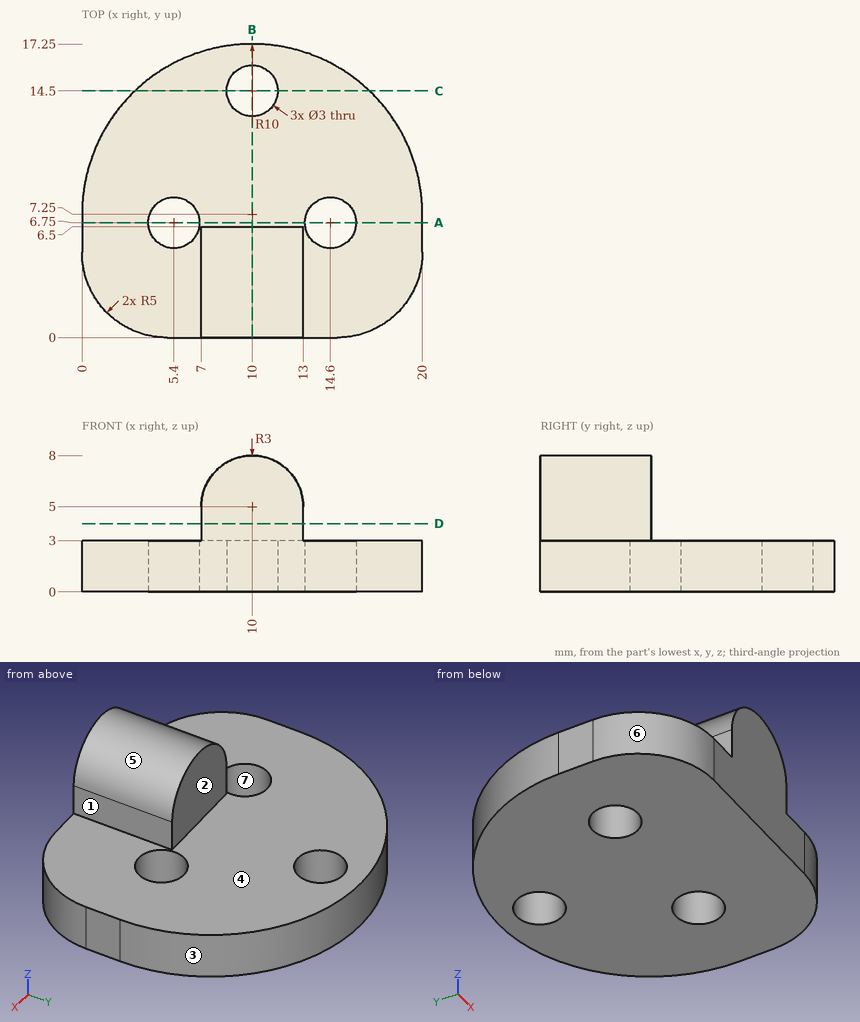
Check sheet for the drawn part. Datum: minimum x, y, z corner. Units: mm. A direction names the side the tool comes from. Coordinates: 2 decimals unless noted, no trailing zeros. Order: outer loops, then holes, each group sorted by start corner. A loop starts at its lowest first (then second) coordinate and runs counter-clockwise, first axis right, second up. Notation, with made-up numbers: (10, 4.5) -> (62, 4.5) arc R20 cw to (62, 8.5) -> close; hole circle Ø3 at (-10, 48.5). An arc over 180 degrees is marked (long way). Use a Markdown table: item, result. Add a question column.
1. Material ranges on L1, parallel to X at y = 6.75, z = 1.45; L2, parallel to Y at x = 10, z = 1.05; L3, parallel to X at y = 5.75, z = 1.75, recorded low to high.
2. Cross-section at A-A (y = 6.75). Enter the section's corners in (x, z), and give its area (3 significant figures).
3. Cross-section at D-D (z = 4). Enter the section's corners in (x, y), and give its area (3 significant figures).
4. Cross-section at B-B (x = 10). Enter the section's corners in (y, z).
5. Set-up check for the marked faces 1, 2 and 3: record each of +Z, -Z, +X, -X, +Y, -Y from which the full face is reachable in a straight line by a thin tool's end or side.
6. Mould release check, pull along X, two halves, no side actions. Record for the marked faces 4, 5, 6 and 7: pulls with the +X half, pulls with the -X half, needs draft (parallel to the pull), parting line crosses it, or undercut.
7. Go/stop test with flat-tipped pins: pin 1 Ø1.5 at (x, y) = (3, 15) entering from +Z; pin 2 Ø1.5 at (x, z) = (11, 4.5) entering from +Y; pin 3 Ø2 at (y, z) = (3.5, 5) entering from +X; pin 4 Ø4 at (x, y) = (8.5, 8) entering from -Z. Record where each tip stops, or that it passes through.
8. Cross-section at C-C (y = 14.5). Enter the section's corners in (x, z), and give its area (3 significant figures).
Filled sheet:
| question | item | result |
|---|---|---|
| 1 | L1 | 0 to 3.9, 6.9 to 13.1, 16.1 to 20 |
| 1 | L2 | 0 to 13, 16 to 17.25 |
| 1 | L3 | 0 to 4.28, 6.52 to 13.48, 15.72 to 20 |
| 2 | outline | (0, 0) -> (3.9, 0) -> (3.9, 3) -> (0, 3) -> close; (6.9, 0) -> (13.1, 0) -> (13.1, 3) -> (6.9, 3) -> close; (16.1, 0) -> (20, 0) -> (20, 3) -> (16.1, 3) -> close |
| 2 | area | 42.0 mm2 |
| 3 | outline | (7, 0) -> (13, 0) -> (13, 6.5) -> (7, 6.5) -> close |
| 3 | area | 39.0 mm2 |
| 4 | outline | (0, 0) -> (13, 0) -> (13, 3) -> (6.5, 3) -> (6.5, 8) -> (0, 8) -> close; (16, 0) -> (17.25, 0) -> (17.25, 3) -> (16, 3) -> close |
| 5 | face 1 | +Z, +X, +Y, -Y |
| 5 | face 2 | +Z, +X, -X, +Y |
| 5 | face 3 | +Z, -Z, +Y |
| 6 | face 4 | needs draft |
| 6 | face 5 | parting line crosses it |
| 6 | face 6 | pulls with the -X half |
| 6 | face 7 | undercut |
| 7 | pin 1 | z = 3 |
| 7 | pin 2 | y = 6.5 |
| 7 | pin 3 | x = 13 |
| 7 | pin 4 | z = 0 |
| 8 | outline | (3.11, 0) -> (8.5, 0) -> (8.5, 3) -> (3.11, 3) -> close; (11.5, 0) -> (16.89, 0) -> (16.89, 3) -> (11.5, 3) -> close |
| 8 | area | 32.3 mm2 |
